```python
from build123d import *

# Parameters (mm, degrees)
F0_W      = 31.8
F0_H      = 15.8
F1_DEPTH  = 4.8
F2_W      = 29.4
F2_H      = 13.4
F3_DEPTH  = 8.4
F4_R      = 2.409
F5_DEPTH  = 1.8
F6_R      = 1.3
F7_DEPTH  = 1.2
F8_R      = 3.255
F8_R_2    = 2.4
F9_DEPTH  = 8.4
F10_W     = 0.3
F10_H     = 0.6
F11_DEPTH = 8.4
F12_W     = 0.6
F12_H     = 0.3
F13_DEPTH = 8.4
F14_W     = 0.8
F14_H     = 3.4696710694
F15_DEPTH = 6.4


with BuildPart() as f1:
    # F0 (on Top) → F1 (new body, symmetric)
    with BuildSketch(Plane.XY):
        Rectangle(F0_W, F0_H)
    extrude(amount=F1_DEPTH, both=True)

    # F2 (on face) → F3 (cut)
    with BuildSketch(Plane(origin=(0, 0, -4.8), x_dir=(1, 0, 0), z_dir=(0, 0, -1))):
        Rectangle(F2_W, F2_H)
    extrude(amount=-F3_DEPTH, mode=Mode.SUBTRACT)

    # F4 (on face) → F5 (join)
    with BuildSketch(Plane.XY.offset(4.8)):
        with Locations((-12, 4)):
            Circle(F4_R)
        with Locations((-4, 4)):
            Circle(F4_R)
        with Locations((-4, -4)):
            Circle(F4_R)
        with Locations((-12, -4)):
            Circle(F4_R)
        with Locations((4, -4)):
            Circle(F4_R)
        with Locations((12, -4)):
            Circle(F4_R)
        with Locations((4, 4)):
            Circle(F4_R)
        with Locations((12, 4)):
            Circle(F4_R)
    extrude(amount=F5_DEPTH)

    # F6 (on face) → F7 (cut)
    with BuildSketch(Plane(origin=(0, 0, 3.6), x_dir=(1, 0, 0), z_dir=(0, 0, -1))):
        with Locations((-12, 4)):
            Circle(F6_R)
        with Locations((-4, 4)):
            Circle(F6_R)
        with Locations((-4, -4)):
            Circle(F6_R)
        with Locations((-12, -4)):
            Circle(F6_R)
        with Locations((4, -4)):
            Circle(F6_R)
        with Locations((12, -4)):
            Circle(F6_R)
        with Locations((4, 4)):
            Circle(F6_R)
        with Locations((12, 4)):
            Circle(F6_R)
    extrude(amount=-F7_DEPTH, mode=Mode.SUBTRACT)

    # F8 (on face) → F9 (join, through all)
    with BuildSketch(Plane(origin=(0, 0, 3.6), x_dir=(1, 0, 0), z_dir=(0, 0, -1))):
        with Locations((-8, 0)):
            Circle(F8_R)
        with Locations((-8, 0)):
            Circle(F8_R_2, mode=Mode.SUBTRACT)
        Circle(F8_R)
        Circle(F8_R_2, mode=Mode.SUBTRACT)
        with Locations((8, 0)):
            Circle(F8_R)
        with Locations((8, 0)):
            Circle(F8_R_2, mode=Mode.SUBTRACT)
    extrude(amount=F9_DEPTH)

    # F10 (on face) → F11 (join, through all)
    with BuildSketch(Plane(origin=(0, 0, 3.6), x_dir=(1, 0, 0), z_dir=(0, 0, -1))):
        with Locations((-14.55, 4)):
            Rectangle(F10_W, F10_H)
        with Locations((-14.55, -4)):
            Rectangle(F10_W, F10_H)
        with Locations((14.55, 4)):
            Rectangle(F10_W, F10_H)
        with Locations((14.55, -4)):
            Rectangle(F10_W, F10_H)
    extrude(amount=F11_DEPTH)

    # F12 (on face) → F13 (join, through all)
    with BuildSketch(Plane(origin=(0, 0, 3.6), x_dir=(1, 0, 0), z_dir=(0, 0, -1))):
        with Locations((-12, 6.55)):
            Rectangle(F12_W, F12_H)
        with Locations((-12, -6.55)):
            Rectangle(F12_W, F12_H)
        with Locations((-4, 6.55)):
            Rectangle(F12_W, F12_H)
        with Locations((-4, -6.55)):
            Rectangle(F12_W, F12_H)
        with Locations((4, 6.55)):
            Rectangle(F12_W, F12_H)
        with Locations((12, 6.55)):
            Rectangle(F12_W, F12_H)
        with Locations((12, -6.55)):
            Rectangle(F12_W, F12_H)
        with Locations((4, -6.55)):
            Rectangle(F12_W, F12_H)
    extrude(amount=F13_DEPTH)

    # F14 (on face) → F15 (join)
    with BuildSketch(Plane(origin=(0, 0, 3.6), x_dir=(1, 0, 0), z_dir=(0, 0, -1))):
        with Locations((0, 4.9651644653)):
            Rectangle(F14_W, F14_H)
        with Locations((0, -4.9651644653)):
            Rectangle(F14_W, F14_H)
    extrude(amount=F15_DEPTH)


solid = f1.part
```
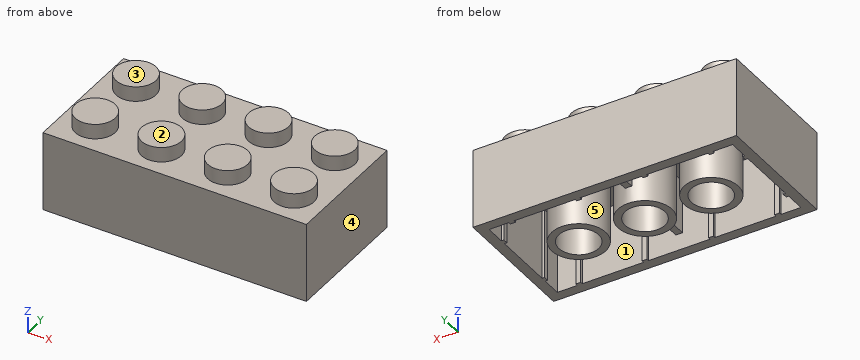
Check sheet for the modelled part. Datum: model origin and axes. Units: mm. Face numbers are marked on the shaded views. A direction names the side the tool comes from. Round coordinates to 2 decimals unless told otherwise and drop trailing zeros. Order: outer loops, then holes, each group sorted by start corner. A loop starts at its lowest first (then second) coordinate and runs counter-clockwise, first axis right, second up. Notation, with made-up numbers: (-12, -3.75) -> (11, -3.75) arc R30 ccw to (11, 18.25) -> close; hole circle Ø10 at (12, -27). An arc over 180 degrees is marked (long way). One line per item, written item: value. Start each with the question number.
Q1. Thickness scan on line 1 (X direction, y = -4, z = 4.15); line 2 (Y direction, x = -12, z = 4); line 3 (Y direction, x = -8, z = -3) (3 decimals). Record the ranges inside material, lowest first.
Q2. Cross-section at A-A (z = 5.75). Record the boundary of the cut face in (x, y), and give its area (3 significant figures).
Q3. Mould release check, pull along X, two halves, no side actions. Record for the marked faces 3, 4 and 5: pulls with the +X half, pulls with the -X half, needs draft (parallel to the pull), parting line crosses it, or undercut.
Q4. Cross-section at C-C (x = 0). Record the boundary of the cut face in (y, z) (3 decimals).
Q5. Gauge pin test, flat ends, axial feed: pin 1 Ø1 at (x, y) = (3, -1) entering from +Z; pin 2 Ø2 at (x, y) = (10.5, 5.5) entering from -Z. Record the tip position at first contact, or that the pin passes through.
Q6. Set-up check for the marked faces 1 and 2: record each of +Z, -Z, +X, -X, +Y, -Y from which the full face is reachable in a straight line by a thin tool's end or side.
Q7. Cross-section at B-B (z = 4). Give the number of separate pieces and of enclosed holes in the cut face, and give its area (3 significant figures).
Completed:
1. line 1: x = -15.9 to -13.3, -10.7 to -5.3, -2.7 to 2.7, 5.3 to 10.7, 13.3 to 15.9
1. line 2: y = -7.9 to -5.3, -2.7 to 2.7, 5.3 to 7.9
1. line 3: y = -7.9 to -6.7, -3.255 to -2.4, 2.4 to 3.255, 6.7 to 7.9
2. outline: circle Ø4.82 at (-12, -4); circle Ø4.82 at (-12, 4); circle Ø4.82 at (-4, -4); circle Ø4.82 at (-4, 4); circle Ø4.82 at (4, -4); circle Ø4.82 at (4, 4); circle Ø4.82 at (12, -4); circle Ø4.82 at (12, 4)
2. area: 146 mm²
3. face 3: needs draft
3. face 4: pulls with the +X half
3. face 5: undercut
4. outline: (-7.9, -4.8) -> (-6.7, -4.8) -> (-6.7, -2.8) -> (-3.255, -2.8) -> (-3.255, -4.8) -> (-2.4, -4.8) -> (-2.4, 3.6) -> (2.4, 3.6) -> (2.4, -4.8) -> (3.255, -4.8) -> (3.255, -2.8) -> (6.7, -2.8) -> (6.7, -4.8) -> (7.9, -4.8) -> (7.9, 4.8) -> (-7.9, 4.8) -> close
5. pin 1: stops at z = 4.8
5. pin 2: stops at z = 3.6
6. face 1: -Z
6. face 2: +Z, +X, -X, +Y, -Y
7. separate pieces: 1
7. enclosed holes: 8
7. area: 460 mm²
